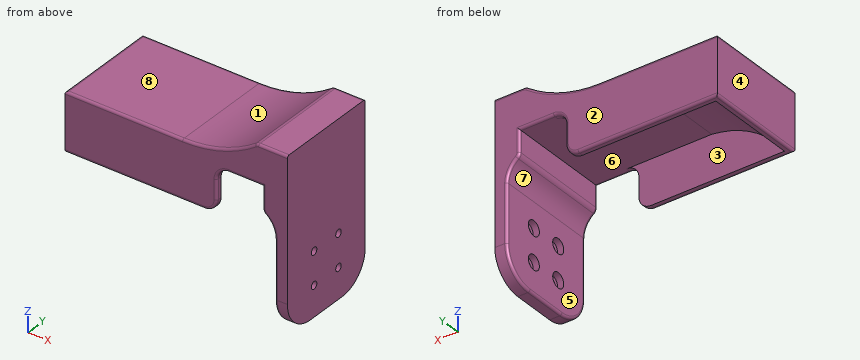
from build123d import *

# Parameters (mm, degrees)
CROQUIS1_W               = 118
CROQUIS1_H               = 84.6
SALIENTE_EXTRUIR1_DEPTH  = 36
CROQUIS2_W               = 36
CROQUIS2_H               = 74.6
CORTAR_EXTRUIR1_DEPTH    = 120
CORTAR_EXTRUIR3_DEPTH    = 110.243581047
SALIENTE_EXTRUIR2_DEPTH  = 84.6
CROQUIS8_W               = 160.5
CROQUIS8_H               = 84.6
SALIENTE_EXTRUIR3_DEPTH  = 5
CROQUIS9_W               = 41
CROQUIS9_H               = 84.6
SALIENTE_EXTRUIR4_DEPTH  = 5
CROQUIS10_W              = 5
CROQUIS10_H              = 84.6
SALIENTE_EXTRUIR5_DEPTH  = 20
REDONDEO2_R              = 10
REDONDEO4_R              = 2
CROQUIS18_W              = 165.5
CROQUIS18_H              = 84.6
SALIENTE_EXTRUIR9_DEPTH  = 6
CROQUIS23_W              = 31
CROQUIS23_H              = 84.6
SALIENTE_EXTRUIR12_DEPTH = 5
CROQUIS19_W              = 120
CROQUIS19_H              = 84.6
SALIENTE_EXTRUIR10_DEPTH = 10
REDONDEO6_R              = 20
REDONDEO9_R              = 5
CROQUIS22_W              = 25
CROQUIS22_H              = 84.6
SALIENTE_EXTRUIR11_DEPTH = 20
REDONDEO7_R              = 100
REDONDEO10_R             = 5
CROQUIS26_R              = 6
CORTAR_EXTRUIR4_DEPTH    = 200.244924653
CROQUIS28_R              = 6
SALIENTE_EXTRUIR14_DEPTH = 5
CROQUIS30_R              = 3
CORTAR_EXTRUIR5_DEPTH    = 195.726834309
REDONDEO11_R             = 25
REDONDEO12_R             = 2
REDONDEO13_R             = 2


with BuildPart() as part:
    # Croquis1 → Saliente-Extruir1 (new body)
    with BuildSketch(Plane.XY):
        Rectangle(CROQUIS1_W, CROQUIS1_H)
    extrude(amount=SALIENTE_EXTRUIR1_DEPTH)

    # Croquis2 → Cortar-Extruir1 (cut)
    with BuildSketch(Plane(origin=(59, 0, 0), x_dir=(0, 0, -1), z_dir=(1, 0, 0))):
        with Locations((-18, 0)):
            Rectangle(CROQUIS2_W, CROQUIS2_H)
    extrude(amount=-CORTAR_EXTRUIR1_DEPTH, mode=Mode.SUBTRACT)


with BuildPart() as cortar_extruir1_piece_1:
    # of the separate pieces the step leaves, piece 1, a body of its own (cortar_extruir1_pieces)
    add(part.part.solids().sort_by_distance((-59, -42.3, 0))[0])


with BuildPart() as cortar_extruir1_piece_2:
    # of the separate pieces the step leaves, piece 2, a body of its own (cortar_extruir1_pieces)
    add(part.part.solids().sort_by_distance((-59, 42.3, 0))[0])


with BuildPart() as cortar_extruir3_tool:
    # Croquis6 → Cortar-Extruir3 (new, through all)
    with BuildSketch(Plane.XZ.offset(42.3)):
        with BuildLine():
            Line((-59, 0), (-59, 36))
            Line((-59, 36), (0, 36))
            ThreePointArc((0, 36), (-33.535731191, 24.614115008), (-59, 0))
        make_face()
    extrude(amount=-CORTAR_EXTRUIR3_DEPTH)


with BuildPart() as cortar_extruir1_piece_1_1:
    add(cortar_extruir1_piece_1.part)

    # Cortar-Extruir3: cut by cortar_extruir3_tool
    add(cortar_extruir3_tool.part, mode=Mode.SUBTRACT)



with BuildPart() as cortar_extruir1_piece_2_1:
    add(cortar_extruir1_piece_2.part)

    # Cortar-Extruir3: cut by cortar_extruir3_tool
    add(cortar_extruir3_tool.part, mode=Mode.SUBTRACT)


with BuildPart() as body_3:
    # Croquis7 → Saliente-Extruir2 (new, through all)
    with BuildSketch(Plane.XZ.offset(-42.3)):
        with BuildLine():
            Line((-59, 0), (-59, 36))
            Line((-59, 36), (0, 36))
            ThreePointArc((0, 36), (-33.535731191, 24.614115008), (-59, 0))
        make_face()
    extrude(amount=SALIENTE_EXTRUIR2_DEPTH)


with BuildPart() as cortar_extruir1_piece_1_2:
    add(cortar_extruir1_piece_1_1.part)

    add(cortar_extruir1_piece_2_1.part)  # Saliente-Extruir3 merges Cortar-Extruir1 piece 2

    add(body_3.part)  # Saliente-Extruir3 merges body 3
    # Croquis8 → Saliente-Extruir3 (add)
    with BuildSketch(Plane.XY.offset(36)):
        with Locations((21.25, 0)):
            Rectangle(CROQUIS8_W, CROQUIS8_H)
    extrude(amount=SALIENTE_EXTRUIR3_DEPTH)

    # Croquis9 → Saliente-Extruir4 (add)
    with BuildSketch(Plane.ZY.offset(59)):
        with Locations((20.5, 0)):
            Rectangle(CROQUIS9_W, CROQUIS9_H)
    extrude(amount=SALIENTE_EXTRUIR4_DEPTH)

    # Croquis10 → Saliente-Extruir5 (add)
    with BuildSketch(Plane(origin=(0, 0, 36), x_dir=(-1, 0, 0), z_dir=(0, 0, -1))):
        with Locations((-99, 0)):
            Rectangle(CROQUIS10_W, CROQUIS10_H)
    extrude(amount=SALIENTE_EXTRUIR5_DEPTH)

    # Redondeo2
    redondeo2_edges = [cortar_extruir1_piece_1_2.edges().sort_by_distance(p)[0] for p in [
        (59, -39.8, 36),
        (59, -39.8, 0),
        (59, 39.8, 36),
        (59, 39.8, 0),
    ]]
    fillet(redondeo2_edges, radius=REDONDEO2_R)

    # Redondeo4
    redondeo4_edges = [cortar_extruir1_piece_1_2.edges().sort_by_distance(p)[0] for p in [
        (-7.5, -42.3, 0),
        (-64, 0, 0),
        (82.75, 42.3, 36),
        (82.75, -42.3, 36),
        (59, -42.3, 18),
        (-7.5, 42.3, 0),
        (56.071067812, -42.3, 2.928932188),
        (59, 42.3, 18),
        (56.071067812, 42.3, 2.928932188),
        (61.928932188, -42.3, 33.071067812),
        (61.928932188, 42.3, 33.071067812),
    ]]
    fillet(redondeo4_edges, radius=REDONDEO4_R)

    # Croquis18 → Saliente-Extruir9 (add)
    with BuildSketch(Plane.XY.offset(41)):
        with Locations((18.75, 0)):
            Rectangle(CROQUIS18_W, CROQUIS18_H)
    extrude(amount=SALIENTE_EXTRUIR9_DEPTH)

    # Croquis23 → Saliente-Extruir12 (add)
    with BuildSketch(Plane(origin=(101.5, 0, 0), x_dir=(0, 0, -1), z_dir=(1, 0, 0))):
        with Locations((-31.5, 0)):
            Rectangle(CROQUIS23_W, CROQUIS23_H)
    extrude(amount=SALIENTE_EXTRUIR12_DEPTH)

    # Croquis19 → Saliente-Extruir10 (add)
    with BuildSketch(Plane(origin=(106.5, 0, 0), x_dir=(0, 0, -1), z_dir=(1, 0, 0))):
        with Locations((13, 0)):
            Rectangle(CROQUIS19_W, CROQUIS19_H)
    extrude(amount=SALIENTE_EXTRUIR10_DEPTH)

    # Redondeo6
    # the kernel refuses this fillet: 20 mm, written as the material it adds along each edge
    with BuildSketch(Plane(origin=(106.5, 42.3, 16), x_dir=(0, 0, -1), z_dir=(0, -1, 0))) as redondeo6_piece_1:
        with BuildLine():
            CenterArc((17.320508076, -20), REDONDEO6_R, 90, 60)
            Line((0, -10), (-0.346410162, -9.8))
            ThreePointArc((-0.346410162, -9.8), (-0.4, -5), (-0.4, 0))
            Line((-0.4, 0), (0, 0.4))
            Line((0, 0.4), (17.320508076, 0.4))
            Line((17.320508076, 0.4), (17.320508076, 0))
        make_face()
    extrude(amount=84.6)

    # Redondeo9
    redondeo9_edges = [cortar_extruir1_piece_1_2.edges().sort_by_distance(p)[0] for p in [
        (96.5, 0, 16),
    ]]
    fillet(redondeo9_edges, radius=REDONDEO9_R)

    # Croquis22 → Saliente-Extruir11 (add)
    with BuildSketch(Plane.XY.offset(47)):
        with Locations((104, 0)):
            Rectangle(CROQUIS22_W, CROQUIS22_H)
    extrude(amount=SALIENTE_EXTRUIR11_DEPTH)

    # Redondeo7
    # the kernel refuses this fillet: 100 mm, written as the material it adds along each edge
    with BuildSketch(Plane(origin=(91.5, 42.3, 47), x_dir=(0, 0, 1), z_dir=(0, -1, 0))) as redondeo7_piece_1:
        with BuildLine():
            CenterArc((100, 60), REDONDEO7_R, 180, 36.869897646)
            Line((0, 60), (-2, 60))
            Line((-2, 60), (-2, 0))
            Line((-2, 0), (0, -2))
            ThreePointArc((0, -2), (10, -2), (18.4, -1.2))
            Line((18.4, -1.2), (20, 0))
        make_face()
    extrude(amount=84.6)

    # Redondeo10
    redondeo10_edges = [cortar_extruir1_piece_1_2.edges().sort_by_distance(p)[0] for p in [
        (91.5, 0, 67),
    ]]
    fillet(redondeo10_edges, radius=REDONDEO10_R)

    # Croquis26 → Cortar-Extruir4 (cut, through all)
    with BuildSketch(Plane(origin=(116.5, 0, 0), x_dir=(0, 0, -1), z_dir=(1, 0, 0))):
        with Locations((21.75, 13.25)):
            Circle(CROQUIS26_R)
        with Locations((48.25, 13.25)):
            Circle(CROQUIS26_R)
        with Locations((48.25, -13.25)):
            Circle(CROQUIS26_R)
        with Locations((21.75, -13.25)):
            Circle(CROQUIS26_R)
    extrude(amount=-CORTAR_EXTRUIR4_DEPTH, mode=Mode.SUBTRACT)

    # Croquis28 → Saliente-Extruir14 (add)
    with BuildSketch(Plane(origin=(116.5, 0, 0), x_dir=(0, 0, -1), z_dir=(1, 0, 0))):
        with Locations((21.75, 13.25)):
            Circle(CROQUIS28_R)
        with Locations((48.25, 13.25)):
            Circle(CROQUIS28_R)
        with Locations((21.75, -13.25)):
            Circle(CROQUIS28_R)
        with Locations((48.25, -13.25)):
            Circle(CROQUIS28_R)
    extrude(amount=-SALIENTE_EXTRUIR14_DEPTH)

    # Croquis30 → Cortar-Extruir5 (cut, through all)
    with BuildSketch(Plane.ZY.offset(-111.5)):
        with Locations((-48.25, 13.25)):
            Circle(CROQUIS30_R)
        with Locations((-21.75, 13.25)):
            Circle(CROQUIS30_R)
        with Locations((-48.25, -13.25)):
            Circle(CROQUIS30_R)
        with Locations((-21.75, -13.25)):
            Circle(CROQUIS30_R)
    extrude(amount=-CORTAR_EXTRUIR5_DEPTH, mode=Mode.SUBTRACT)

    # Redondeo11
    redondeo11_edges = [cortar_extruir1_piece_1_2.edges().sort_by_distance(p)[0] for p in [
        (111.5, -42.3, -73),
        (111.5, 42.3, -73),
    ]]
    fillet(redondeo11_edges, radius=REDONDEO11_R)

    # Redondeo12
    redondeo12_edges = [cortar_extruir1_piece_1_2.edges().sort_by_distance(p)[0] for p in [
        (106.5, -42.3, -24.660254038),
        (104.38854382, 42.3, 7.623763834),
        (104.38854382, -42.3, 7.623763834),
        (96.5, 42.3, 28.339745962),
        (97.027864045, 42.3, 16.443423947),
        (96.5, -42.3, 28.339745962),
        (97.027864045, -42.3, 16.443423947),
        (106.5, 0, -73),
        (106.5, 42.3, -24.660254038),
        (106.5, 34.97766953, -65.67766953),
        (106.5, -34.97766953, -65.67766953),
    ]]
    fillet(redondeo12_edges, radius=REDONDEO12_R)

    # Redondeo13
    redondeo13_edges = [cortar_extruir1_piece_1_2.edges().sort_by_distance(p)[0] for p in [
        (-64, 0, 47),
        (-16.25, -42.3, 47),
        (104.822070015, 42.3, 67),
        (-16.25, 42.3, 47),
        (62.360669992, 42.3, 51.881026879),
        (104.822070015, -42.3, 67),
        (62.360669992, -42.3, 51.881026879),
        (91.60110653, -42.3, 66.755948656),
        (91.60110653, 42.3, 66.755948656),
    ]]
    fillet(redondeo13_edges, radius=REDONDEO13_R)


solid = cortar_extruir1_piece_1_2.part
The listing builds one solid part. Answer for the finished solid, in the listing's coordinates (mm). Face numbers are marked on the shaded views. A direction names the side the tool comes from. Round coordinates to 2 decimals unless told otherwise and drop trailing zeros. Write each loop counter-clockwise with the first axis right and the second up, starting at its lowest first coordinate (ties: lowest second). Pieces come first, ordered by that corner, then holes. Notation, with made-up numbers: M 7,-4 L 32,-4 A19 ccw 32,5 Z; hole C -27,50.25 d5. An arc over 180 degrees is marked long. Write each question's results on one line, items separated by ' | '. Start each with the question number.
(1) The part is cut by section C-C, the plane y = -1. Write down the section's boundary in (x, z).
(2) The part is cut by section D-D, the plane x = -50. Write down the section's boundary in (y, z).
(3) The part is cut by section A-A, the plane z = -21.75. Write down the section's boundary in (x, y).
(4) For the marked faces 4, 5, 6, 7 and 8, determine the directions among +Z, -Z, +X, -X, +Y, -Y from which every point of the face is accessible in a straight line to the end or side of a thin tool.
(5) Each of these flat-tipped pins is pushed along its axis until it touches: P1, Ø15.5, axis at y = 13.25, z = -21.75, coming from the -X side; P2, Ø6, axis at x = -18.5, y = 15.5, coming from the +Z side; P3, Ø1.5, axis at x = 10.5, y = 11.5, coming from the -Z side; P4, Ø15.5, axis at y = -13.25, z = -21.75, coming from the +X side. Where does it stop, or does it pass through?
(6) The part is cut by section B-B, the plane y = -13.25. Give the number of separate pieces and of enclosed holes in the cut face, and give its area (3 significant figures).
(7) Find the intervals of material crossed by line 1 (Y direction, x = 114, z = -48); line 2 (Y direction, x = 108.1, z = -21.75); line 3 (Z direction, x = 115, y = -13), in increasing order.
(8) Determine the mould class of the marked faces 1, 2 and 3 for opening direction X: +X half, -X half, draft (parallel to the pull), parting line (faces both ways), or undercut.
Worked answers:
1) outline: M -64,2 A2 ccw -62,0 L -59,0 A80.94 cw 0,36 L 96.5,36 L 96.5,18.68 A5 ccw 98.5,14.68 A20 cw 106.5,-1.32 L 106.5,-71 A2 ccw 108.5,-73 L 116.5,-73 L 116.5,67 L 93.14,67 A5 ccw 90.21,66.05 A100 cw 31.5,47 L -62,47 A2 ccw -64,45 Z
2) outline: M -42.3,2 A2 ccw -40.3,0 L -37.3,0 L -37.3,11.33 L 37.3,11.33 L 37.3,0 L 40.3,0 A2 ccw 42.3,2 L 42.3,45 A2 ccw 40.3,47 L -40.3,47 A2 ccw -42.3,45 Z
3) outline: M 106.5,-40.3 A2 ccw 108.5,-42.3 L 116.5,-42.3 L 116.5,-16.25 L 111.5,-16.25 L 111.5,-19.25 L 106.5,-19.25 Z; M 106.5,-7.25 L 111.5,-7.25 L 111.5,-10.25 L 116.5,-10.25 L 116.5,10.25 L 111.5,10.25 L 111.5,7.25 L 106.5,7.25 Z; M 106.5,19.25 L 111.5,19.25 L 111.5,16.25 L 116.5,16.25 L 116.5,42.3 L 108.5,42.3 A2 ccw 106.5,40.3 Z
4) face 4: +Z, -Z, -X, +Y, -Y | face 5: -Z, -X, +Y, -Y | face 6: -Z | face 7: -Z, +Y, -Y | face 8: +Z, -X, +Y, -Y
5) P1: stops at x = 106.5 | P2: stops at z = 47 | P3: stops at z = 36 | P4: stops at x = 116.5
6) separate pieces: 3 | enclosed holes: 0 | area: 4,910 mm²
7) line 1: y = -42.3 to -16.24, -10.26 to 10.26, 16.24 to 42.3 | line 2: y = -42.26 to -19.25, -7.25 to 7.25, 19.25 to 42.26 | line 3: z = -73 to -51.24, -45.26 to -24.74, -18.76 to 67
8) face 1: -X half | face 2: draft | face 3: undercut
